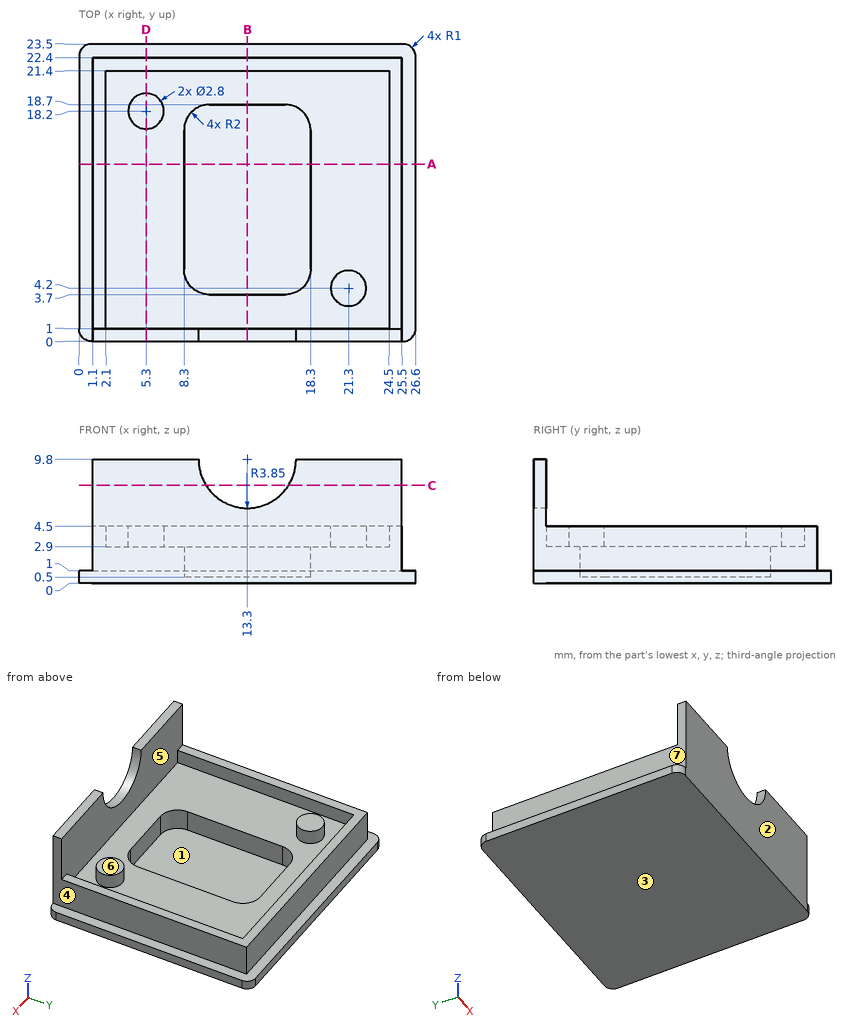
Input: dimensioned drawing with shaded views. Units: mm. Origin: part minimum x, y, z. A direction names the side the tool comes from. Give positions to 0.01 mm unless a question says otherwise; leave off trailing zeros. Write each loop counter-clockwise with the first axis right and the second up, starting at its lowest first coordinate (ties: lowest second). Pieces come first, ordered by that corner, then holes. Notation, with made-up numbers: (42, -21) -> (85, -21) arc R23 ccw to (85, 16) -> close; hole circle Ø11 at (44.25, 85). An arc over 180 degrees is marked (long way). Answer as a JSON object with one key per item and string values.
1. Cut plane C-C on z = 7.75. Output: boundary loops of the cut face in (x, y).
Ans:
{"outline": "(1.1, 0) -> (10.04, 0) -> (10.04, 1) -> (1.1, 1) -> close; (16.56, 0) -> (25.5, 0) -> (25.5, 1) -> (16.56, 1) -> close"}
2. Cut plane A-A on y = 14. Output: boundary loops of the cut face in (x, z), and give its area (3 significant figures).
Ans:
{"outline": "(0, 0) -> (26.6, 0) -> (26.6, 1) -> (25.5, 1) -> (25.5, 4.5) -> (24.5, 4.5) -> (24.5, 2.9) -> (18.3, 2.9) -> (18.3, 0.5) -> (8.3, 0.5) -> (8.3, 2.9) -> (2.1, 2.9) -> (2.1, 4.5) -> (1.1, 4.5) -> (1.1, 1) -> (0, 1) -> close", "area": "52.2 mm^2"}
3. Mould query, pull axis Y, two halves, no side actions, for the marked faces 1, 2 and 3. Classes: pulls with the +Y half, pulls with the -Y half, needs draft (parallel to the pull), parting line crosses it, or undercut.
Ans:
{"face 1": "undercut", "face 2": "pulls with the -Y half", "face 3": "needs draft"}
4. Access query for the marked faces 4, 5, 6 and 7. Directions: +Z, -Z, +X, -X, +Y, -Y. A direction counts if a zero-diameter tool reaches every point of the face in a straight line with its end or side. Return the directions, or none.
Ans:
{"face 4": "+Z, +X, +Y, -Y", "face 5": "+Z", "face 6": "+Z, +X, -X, +Y", "face 7": "+Z, -X, +Y, -Y"}
5. Ray query, probe 1 along X at (y, z) = (8.25, 3.75); probe 2 along X at (y, z) = (7.25, 2.75); probe 3 along Y at (x, z) = (1.5, 2.25). Return the intervals inside material, ascending. Write a range as from..to.
Ans:
{"probe 1": "x = 1.1..2.1, 24.5..25.5", "probe 2": "x = 1.1..8.3, 18.3..25.5", "probe 3": "y = 0..22.4"}
6. Contact query for flat-ended pins moving along their axis: pin 1 (2 mm diameter, centred on y = 14, z = 4.5, fed in from +X); pin 2 (0.7 mm diameter, centred on y = 10, z = 1.5, fed in from -X); pin 3 (8 mm diameter, centred on x = 22.5, y = 18.5, fed in from +Z). Output: stop coordinate, or through.
Ans:
{"pin 1": "stops at x = 25.5", "pin 2": "stops at x = 1.1", "pin 3": "stops at z = 4.5"}
7. Cut plane D-D on x = 5.3. Output: boundary loops of the cut face in (y, z).
Ans:
{"outline": "(0, 0) -> (23.5, 0) -> (23.5, 1) -> (22.4, 1) -> (22.4, 4.5) -> (21.4, 4.5) -> (21.4, 2.9) -> (19.6, 2.9) -> (19.6, 4.5) -> (16.8, 4.5) -> (16.8, 2.9) -> (1, 2.9) -> (1, 9.8) -> (0, 9.8) -> close"}
8. Cut plane B-B on x = 13.3. Output: boundary loops of the cut face in (y, z).
Ans:
{"outline": "(0, 0) -> (23.5, 0) -> (23.5, 1) -> (22.4, 1) -> (22.4, 4.5) -> (21.4, 4.5) -> (21.4, 2.9) -> (18.7, 2.9) -> (18.7, 0.5) -> (3.7, 0.5) -> (3.7, 2.9) -> (1, 2.9) -> (1, 5.95) -> (0, 5.95) -> close"}
